from build123d import *

# Parameters (mm, degrees)
ESQUISSE1_W             = 20
ESQUISSE1_H             = 20
BOSS_EXTRU_1_DEPTH      = 5
ESQUISSE2_W             = 5
ESQUISSE2_H             = 20
BOSS_EXTRU_2_DEPTH      = 70
ESQUISSE3_W             = 20
ESQUISSE3_H             = 20
BOSS_EXTRU_3_DEPTH      = 5
ESQUISSE4_W             = 3
ESQUISSE4_H             = 0.6
ENL_V_MAT_EXTRU_1_DEPTH = 90
ESQUISSE5_W             = 80
ESQUISSE5_H             = 0.25
BOSS_EXTRU_4_DEPTH      = 0.5
ESQUISSE8_W             = 10
ESQUISSE8_H             = 20
BOSS_EXTRU_6_DEPTH      = 10
BOSS_EXTRU_8_DEPTH      = 0.125
BOSS_EXTRU_8_DEPTH_BACK = 0.125


with BuildPart() as part:
    # Esquisse1 → Boss.-Extru.1 (new body)
    with BuildSketch(Plane.XY):
        Rectangle(ESQUISSE1_W, ESQUISSE1_H)
    extrude(amount=BOSS_EXTRU_1_DEPTH)

    # Esquisse2 → Boss.-Extru.2 (add)
    with BuildSketch(Plane.XY.offset(5)):
        with Locations((7.5, 0)):
            Rectangle(ESQUISSE2_W, ESQUISSE2_H)
    extrude(amount=BOSS_EXTRU_2_DEPTH)

    # Esquisse3 → Boss.-Extru.3 (add)
    with BuildSketch(Plane.XY.offset(75)):
        Rectangle(ESQUISSE3_W, ESQUISSE3_H)
    extrude(amount=BOSS_EXTRU_3_DEPTH)

    # Esquisse4 → Enlèv. mat.-Extru.1 (cut)
    with BuildSketch(Plane.XY.offset(80)):
        with Locations((-8.5, 0)):
            Rectangle(ESQUISSE4_W, ESQUISSE4_H)
    extrude(amount=-ENL_V_MAT_EXTRU_1_DEPTH, mode=Mode.SUBTRACT)

    # Esquisse5 → Boss.-Extru.4 (add)
    with BuildSketch(Plane.ZY.offset(7)):
        with Locations((40, 0)):
            Rectangle(ESQUISSE5_W, ESQUISSE5_H)
    extrude(amount=BOSS_EXTRU_4_DEPTH)

    # Esquisse8 → Boss.-Extru.6 (add)
    with BuildSketch(Plane(origin=(10, 0, 0), x_dir=(0, 0, -1), z_dir=(1, 0, 0))):
        with Locations((-40, 0)):
            Rectangle(ESQUISSE8_W, ESQUISSE8_H)
    extrude(amount=BOSS_EXTRU_6_DEPTH)

    # Esquisse10 → Boss.-Extru.8 (add, two sides: drawn at the far end of the back side and taken through both)
    with BuildSketch(Plane(origin=(0, 0, 0), x_dir=(1, 0, 0), z_dir=(0, 1, 0)).offset(-BOSS_EXTRU_8_DEPTH_BACK)):
        Polygon((10, -79.5), (19.7, -45), (20, -45), (10, -80), align=None)
        Polygon((19.7, -35), (20, -35), (10, 0), (10, -0.5), align=None)
    extrude(amount=BOSS_EXTRU_8_DEPTH + BOSS_EXTRU_8_DEPTH_BACK)


solid = part.part
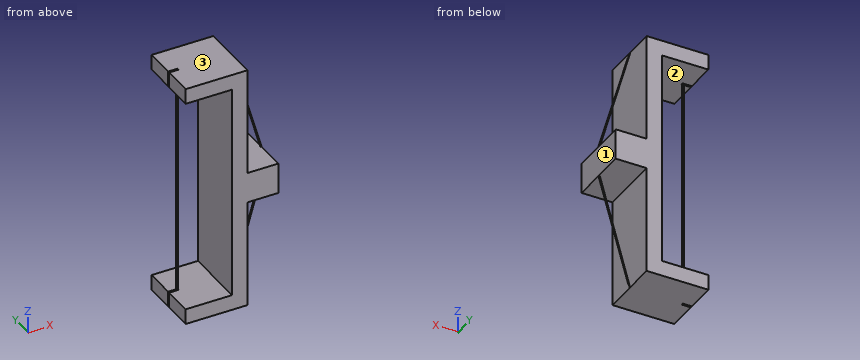
Can you work these out from the model? Positions are in its coordinate system, mm. Face numbers are marked on the shaded views. Give positions to 0.01 mm unless a question says otherwise; leave off trailing zeros. Loops run counter-clockwise (first coordinate to the right, second up) from the corner with the lowest first, then second, coordinate; pieces in that order, holes last. Notation, with made-up numbers: (77, 42.5) -> (111, 42.5) arc R29 ccw to (111, 73.5) -> close; hole circle Ø5 at (36, -19.75). An arc over 180 degrees is marked (long way). Write item = value, one per line.
1) Thinking about a two-plate mould opening in Z: for the marked faces 1, 2 and 3, which applies, released by +Z, released by -Z, zero draft, split by the parting line, or undercut?
Check result:
face_1 = zero draft
face_2 = undercut
face_3 = released by +Z
2) Will these pins go through, and if not, where does the flat tip stop? pin 1 (8 mm diameter, centred on y = 1.5, z = 14.5, fed in from -X); pin 2 (3 mm diameter, centred on x = 13, z = 60, fed in from +Y); pin 3 (1 mm diameter, centred on y = 4.5, z = 20.5, fed in from -X).
Check result:
pin_1 = -7.5
pin_2 = through
pin_3 = 5
3) Suppose I cut it at C-C on y = -5.25. Write out the boundary of the cut face in (x, z), then the cut area to 3 significant figures.
Check result:
outline = (-10, 0) -> (10, 0) -> (10, 35) -> (20, 35) -> (20, 45) -> (10, 45) -> (10, 80) -> (-10, 80) -> (-10, 75) -> (5, 75) -> (5, 5) -> (-10, 5) -> close
area = 650 mm2
4) Suppose I cut it at D-D on z = 15.5. Write out the boundary of the cut face in (x, y) (3 decimals), then the cut area to 3 significant figures.
Check result:
outline = (-7.5, -0.125) -> (-7, -0.125) -> (-7, 0.125) -> (-7.5, 0.125) -> close; (5, -10) -> (10, -10) -> (10, 10) -> (5, 10) -> close; (14.217, -0.125) -> (14.429, -0.125) -> (14.429, 0.125) -> (14.217, 0.125) -> close
area = 100 mm2
5) Suppose I cut it at B-B on x = -3.5. Write out the boundary of the cut face in (y, z).
Check result:
outline = (-10, 0) -> (10, 0) -> (10, 5) -> (-10, 5) -> close; (-10, 75) -> (10, 75) -> (10, 80) -> (-10, 80) -> close
6) I need wall thicknesses on L1, parallel to Z at x = -6.5, y = 6.75; L2, parallel to X at y = 8.25, z = 32.5; L3, parallel to Z at x = 18.25, y = 1.75. Which ranges of each line are inside material? Lowest first, please. Write a range as from..to.
Check result:
L1 = 0..5, 75..80
L2 = 5..10
L3 = 35..45
7) Suppose I cut it at A-A on z = 44. Write out the boundary of the cut face in (x, y) (3 decimals), then the cut area to 3 significant figures.
Check result:
outline = (-7.5, -0.125) -> (-7, -0.125) -> (-7, 0.125) -> (-7.5, 0.125) -> close; (5, -10) -> (20, -10) -> (20, 10) -> (5, 10) -> close
area = 300 mm2
